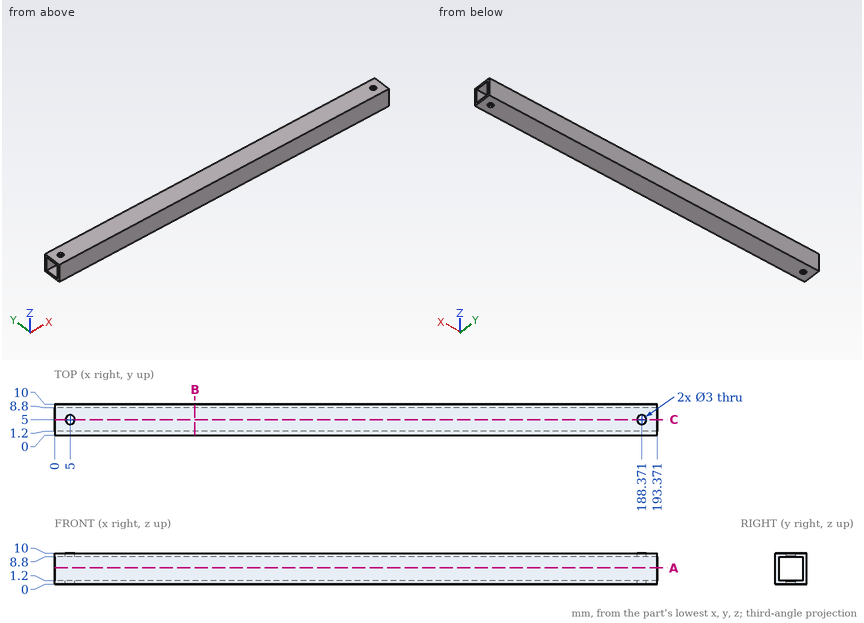
Check sheet for the drawn part. Datum: minimum x, y, z corner. Units: mm. Round coordinates to 2 decimals unless told otherwise and drop trailing zeros. Loops run counter-clockwise (first coordinate to the right, second up) from the corner with the lowest first, then second, coordinate; pieces in that order, holes last. Notation, with made-up numbers: (4, 85.25) - (30, 85.25) arc R16 cw to (30, 105.25) - close; hole circle Ø4 at (-3, 9). An arc over 180 degrees is marked (long way). Write each question's results on one line, items separated by ' | '. Start each with the question number.
Q1. Cross-section at B-B on x = 45. Enter the section's corners in (y, z).
Q2. Thickness scan on line 1 (X direction, y = 5, z = 0.65); line 2 (Z direction, x = 87, y = 4.5). Record the ranges inside material, lowest first. Write a range as [from, to].
Q3. Cross-section at C-C on y = 5. Enter the section's corners in (x, z).
Q4. Cross-section at A-A on z = 5.25. Enter the section's corners in (x, y).
Q5. Gauge pin test, flat end, axial feed: P1, Ø5, axis at x = 188.37, y = 5, coming from the -Z side. Record the tip position at first contact, or that the pin passes through.
Answers below:
1) outline: (0, 0) - (10, 0) - (10, 10) - (0, 10) - close; hole (1.2, 1.2) - (8.8, 1.2) - (8.8, 8.8) - (1.2, 8.8) - close
2) line 1: x = [0, 3.5], [6.5, 186.87], [189.87, 193.37] | line 2: z = [0, 1.2], [8.8, 10]
3) outline: (0, 0) - (3.5, 0) - (3.5, 1.2) - (0, 1.2) - close; (0, 8.8) - (3.5, 8.8) - (3.5, 10) - (0, 10) - close; (6.5, 0) - (186.87, 0) - (186.87, 1.2) - (6.5, 1.2) - close; (6.5, 8.8) - (186.87, 8.8) - (186.87, 10) - (6.5, 10) - close; (189.87, 0) - (193.37, 0) - (193.37, 1.2) - (189.87, 1.2) - close; (189.87, 8.8) - (193.37, 8.8) - (193.37, 10) - (189.87, 10) - close
4) outline: (0, 0) - (193.37, 0) - (193.37, 1.2) - (0, 1.2) - close; (0, 8.8) - (193.37, 8.8) - (193.37, 10) - (0, 10) - close
5) P1: stops at z = 0
